Can you work these out from the model? Positions are in its coordinate system, mm. A direction names the side the tool comes from. Give positions to 0.01 mm unless a question says otherwise; leave off trailing zeros. Loops run counter-clockwise (first coordinate to the right, second up) from the corner with the lowest first, then second, coordinate; pieces in that order, holes last. Notation, with made-up numbers: (38.25, 50) - (47.25, 50) arc R25 ccw to (47.25, 81) - close; hole circle Ø5 at (57, 47.25). An arc over 180 degrees is marked (long way). Use a Markdown table: item, result. Add a question column.
Autodesk Inventor part; units mm, degrees
ref_plane "MSC_PF1" through (0, 0, 0) normal (1, 0, 0) x (0, 1, 0)
ref_plane "MSC_PT1" through (0, 0, 0) normal (0, 0, -1) x (-1, 0, 0)
ref_plane "YZ Plane" through (0, 0, 0) normal (1, 0, 0) x (0, 1, 0)
sketch "Esquisse1" plane through (0, 0, 0) normal (0, 1, 0) x (-1, 0, 0)
  point P0 (0, 0)
sketch "Esquisse2" plane through (0, 0, 0) normal (0, 0, 1) x (1, 0, 0)
  point P0 (0, 0)
sketch "Esquisse3" plane through (0, 0, 0) normal (0, 0, 1) x (1, 0, 0)
  point P0 (0, 0)
sketch "Esquisse4" plane through (0, 0, 0) normal (0, 1, 0) x (-1, 0, 0)
  line L0 (-2.75, 0) -> (0, 0)
  line L1 (-2.75, -0.4) -> (-2.75, 0)
  line L2 (-1.5, -1.65) -> (-2.75, -0.4)
  line L3 (-1.5, -1.9) -> (-1.5, -1.65)
  line L4 (-1.25, -2.15) -> (-1.5, -1.9)
  line L5 (-1.5, -2.4) -> (-1.25, -2.15)
  line L6 (-1.5, -14) -> (-1.5, -2.4)
  line L7 (0, 0) -> (0, -14)
  line L8 (0, 3.3392) -> (0, -10.7) construction
  line L9 (0, 3.3392) -> (0, -10.7)
  line L10 (0, -17.4678) -> (0, 6.8071)
  line L11 (-1.5, -14) -> (0, -14)
  line L12 (0.55, 0) -> (-3.3, 0)
  dimension "d3" = 2.75
  dimension "d5" = 0.25
  dimension "d7" = 0.25
  dimension "d9" = 0.25
  dimension "d11" = 1.65
  dimension "d13" = 135
  dimension "d17" = 1.25
  dimension "d19" = 0
  dimension "d51" = 1.5
  dimension "d52" = 14
revolve "Révolution1" add sketch "Esquisse4" angle 360 about axis through (0, 0, 3.3392) along (0, 0, -1)
sketch "Esquisse5" plane through (0, 0, 0) normal (0, 1, 0) x (-1, 0, 0)
  line L0 (-1.6, 0) -> (0, 0)
  line L1 (-0.2667, -1.5) -> (-1.6, 0)
  line L2 (0, -1.5) -> (-0.2667, -1.5)
  line L3 (0, 0) -> (0, -1.5)
  line L4 (-1.5, -1.65) -> (1.5, -1.65) construction
  line L5 (-2.75, 0) -> (2.75, 0)
  line L6 (0, -1.98) -> (0, 0.33)
  dimension "d22" = 1.6
  dimension "d24" = 0.2667
  dimension "d26" = 1.5
extrude "Extrusion1" cut sketch "Esquisse5" along normal mid plane 0.5333
pattern_circular "RéseauPolaire1" count 4 over 360 about axis through (0, 0, 0) along (0, 0, 1) of "Extrusion1"
sketch "Esquisse7" plane through (0, 0, 0) normal (0, 1, 0) x (-1, 0, 0)
  line L0 (0, -0.825) -> (-2, 0)
  line L1 (0, 0) -> (0, -0.825)
  line L2 (-2, 0) -> (0, 0)
  line L3 (-1.5, -1.65) -> (1.5, -1.65) construction
  line L4 (0, -1.98) -> (0, 0.33)
  line L5 (-2.75, 0) -> (2.75, 0)
  dimension "d33" = 2
  dimension "d35" = 0.825
extrude "Extrusion2" cut sketch "Esquisse7" along normal mid plane 0.5333
pattern_circular "RéseauPolaire2" count 4 over 360 about axis through (0, 0, 0) along (0, 0, 1) of "Extrusion2"
fillet "Congé1" radius 0.5 1 edges at (-1.5, 0, -1.65)
thread "Filetage1"
ref_plane "MSC_PF1" through (0, 0, 0) normal (1, 0, 0) x (0, 1, 0)
ref_plane "MSC_PT1" through (0, 0, 0) normal (0, 0, -1) x (-1, 0, 0)
equation "\"d3\" = 0.5 * Dh"
equation "\"d5\" = msp_x"
equation "\"d7\" = ParA"
equation "\"d9\" = msp_x"
equation "\"d11\" = ParK"
equation "\"d17\" = 0.5 * msp_mdtds"
equation "\"d51\" = 0.5 * NND"
equation "\"d52\" = NLG"
equation "\"d22\" = 0.5 * M"
equation "\"d24\" = 0.0833333 * M"
equation "\"d26\" = 0.909091 * ParK"
equation "\"d27\" = 0.166667 * M"
equation "\"d33\" = 0.625 * M"
equation "\"d35\" = 0.5 * ParK"
equation "\"d36\" = 0.166667 * M"
equation "\"d41\" = 2 * msp_x"
equation "\"PTC\" = 0.5"
equation "\"NLG\" = 14"
equation "\"ParK\" = 1.65"
equation "\"NND\" = 3"
equation "\"M\" = 3.2"
equation "\"msp_mdtds\" = NND - PTC"
equation "\"Dh\" = 5.5"
equation "\"msp_x\" = 0.5 * PTC"
equation "\"ParA\" = 0.5 * PTC"
equation "\"r\" = 0.8"
equation "\"THREADDIA\" = NND"
equation "\"TEMPLATE\" = 1.2345"
properties part number "NF EN ISO 7046-2 H - M3x14 - 8.8 - H1" material "Acier inoxydable 440C"
1. Suppose I cut it at A-A (z = -6.75). List the corners of the cut face in (x, y) for me, and give its area (3 significant figures).
2. Please list where these lines run through material, in increasing order: line 1 along Z through (x, y) = (1.5, 1.1); line 2 along Z through (x, y) = (0.5, 0.1); line 3 along X through (y, z) = (-1, -9.25). Write a range as [from, to].
3. If we mould it in two halves opening along Y, with no side actions, what happens to faces 3 (the face through (0.267, -0.8, -0.4)), 4 (the face through (-0.596, -2.685, -0.197)), 5 (the face through (0, 0, -14))? For each: released by +Y, released by -Y, zero draft, split by the parting line, or undercut.
4. Will these pins go through, and if not, where does the flat tip stop? P1, Ø2, axis at x = -1, z = -4, coming from the +Y side; P2, Ø0.8, axis at y = 1, z = -0.5, coming from the +X side; P3, Ø1.2, axis at y = -1.5, z = -0.5, coming from the -X side.
5. On a 3-axis mill with a long thin cutter (end or side, diameter ignored), from which of +Z, -Z, +X, -X, +Y, -Y can I reach the whole of each face in a straight line? I mean faces 1 (the face through (-0.267, 0.8, -0.4)), 2 (the face through (-1.5, 0.07, -8.12)). Say none if no direction works.
Results below:
| question | item | result |
|---|---|---|
| 1 | outline | circle Ø3 at (0, 0) |
| 1 | area | 7.07 mm² |
| 2 | line 1 | [-1.29, 0] |
| 2 | line 2 | [-14, -1.24] |
| 2 | line 3 | [-1.12, 1.12] |
| 3 | face 3 | undercut |
| 3 | face 4 | split by the parting line |
| 3 | face 5 | zero draft |
| 4 | P1 | y = 1.5 |
| 4 | P2 | x = 2.68 |
| 4 | P3 | x = -2.6 |
| 5 | face 1 | +Z |
| 5 | face 2 | -Z |
